from build123d import *

# Parameters (mm, degrees)
F0_R     = 1
F1_DEPTH = 2
F2_R     = 1
F3_DEPTH = 6


# Not quite as in the source:
# - a feature of the source that left no trace in its solid (it failed there, or was rolled back) is left out


with BuildPart() as f1:
    # F0 (on Front) → F1 (new body)
    with BuildSketch(Plane.XZ):
        Polygon((-2, 1.1547005384), (-2, -1.1547005384), (0, -2.3094010768), (2, -1.1547005384), (2, 1.1547005384), (0, 2.3094010768), align=None)
        Circle(F0_R, mode=Mode.SUBTRACT)
        Circle(F0_R)
    extrude(amount=F1_DEPTH)

    # F2 (on face) → F3 (join)
    with BuildSketch(Plane(origin=(0, 0, 0), x_dir=(-1, 0, 0), z_dir=(0, 1, 0))):
        Circle(F2_R)
    extrude(amount=F3_DEPTH)


solid = f1.part
Check sheet for the modelled part. Datum: model origin and axes. Units: mm. A direction names the side the tool comes from. Round coordinates to 2 decimals unless told otherwise and drop trailing zeros. Order: outer loops, then holes, each group sorted by start corner. A loop starts at its lowest first (then second) coordinate and runs counter-clockwise, first axis right, second up. Notation, with made-up numbers: M -4,70.25 L 1,70.25 A34 cw 1,101.25 Z; hole C 49.5,78 d10. An arc over 180 degrees is marked long. One line per item, written item: value. Start each with the question number.
1. Section check A-A on z = 0. Enter the section's corners in (x, y), and give its area (3 significant figures).
2. Section check D-D on y = -1. Enter the section's corners in (x, z), and give its area (3 significant figures).
3. Section check C-C on y = 3.5. Enter the section's corners in (x, z).
4. Release check for a two-part mould opening along Y. For faces 1 (the flat face through (0, 6, 0)), 2 (the flat face through (0, -2, 0)), 3 (the cylindrical face through (0, 3, -1)) record: released by +Y, released by -Y, zero draft, split by the parting line, or undercut.
5. Access from +Z, -Z, +X, -X, +Y, -Y to the whole of each face (thin tool, end or side, straight path). Record for faces 4 (the flat face through (-2, -1, 0)), 5 (the flat face through (-1, 0, 1)).
6. Section check B-B on x = -0.9. Enter the section's corners in (y, z).
7. Scan lines: line 1 along Y through (x, z) = (-1.25, 1); line 2 along Z through (x, y) = (-1.2, -1); line 3 along Z through (x, y) = (1.65, -0.5). Record each from-to range of solid material in increasing order.
Results found:
1. outline: M -2,-2 L 2,-2 L 2,0 L 1,0 L 1,6 L -1,6 L -1,0 L -2,0 Z
1. area: 20.0 mm^2
2. outline: M -2,-1.15 L 0,-2.31 L 2,-1.15 L 2,1.15 L 0,2.31 L -2,1.15 Z
2. area: 13.9 mm^2
3. outline: C 0,0 d2
4. face 1: released by +Y
4. face 2: released by -Y
4. face 3: zero draft
5. face 4: +Z, -Z, -X, +Y, -Y
5. face 5: +Y
6. outline: M -2,-1.79 L 0,-1.79 L 0,-0.44 L 6,-0.44 L 6,0.44 L 0,0.44 L 0,1.79 L -2,1.79 Z
7. line 1: -2 to 0
7. line 2: -1.62 to 1.62
7. line 3: -1.36 to 1.36
